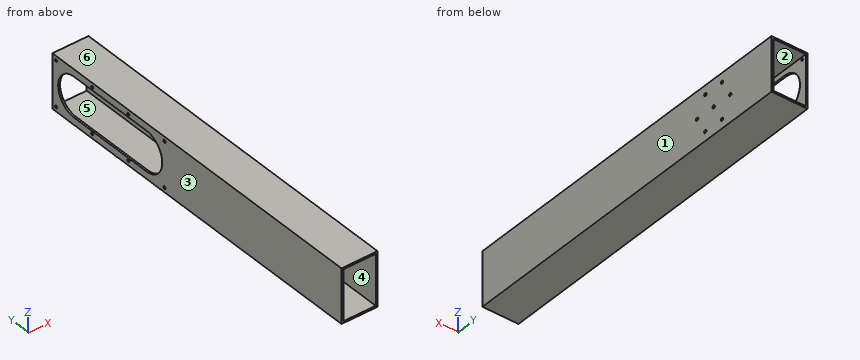
from build123d import *

# Parameters (mm, degrees)
SKETCH1_W                         = 40
SKETCH1_H                         = 60
SKETCH1_W_2                       = 36
SKETCH1_H_2                       = 56
BOSS_EXTRUDE1_DEPTH               = 400
M3_CLEARANCE_HOLE1_D              = 3.4
CUT_EXTRUDE1_DEPTH                = 3
TAP_DRILL_FOR_M3_TAP1_D           = 2.5
TAP_DRILL_FOR_M3_TAP1_DEPTH       = 2
TAP_DRILL_FOR_M3_TAP1_CSINK_D     = 3
TAP_DRILL_FOR_M3_TAP1_CSINK_ANGLE = 90


with BuildPart() as part:
    # Sketch1 → Boss-Extrude1 (new body)
    with BuildSketch(Plane(origin=(0, 0, 0), x_dir=(1, 0, 0), z_dir=(0, 1, 0))):
        with Locations((20, 30)):
            Rectangle(SKETCH1_W, SKETCH1_H)
        with Locations((20, 30)):
            Rectangle(SKETCH1_W_2, SKETCH1_H_2, mode=Mode.SUBTRACT)
    extrude(amount=BOSS_EXTRUDE1_DEPTH)

    # M3 Clearance Hole1 (through all)
    with Locations(Plane(origin=(40, 0, 0), x_dir=(0, 0, -1), z_dir=(1, 0, 0))):
        with Locations((30, 320), (30, 343), (49.918584287, 331.5), (49.918584287, 308.5), (30, 297), (10.081415713, 308.5), (10.081415713, 331.5)):
            Hole(M3_CLEARANCE_HOLE1_D / 2)

    # Sketch4 → Cut-Extrude1 (cut)
    with BuildSketch(Plane.ZY):
        with BuildLine():
            Line((-52, 270), (-52, 370))
            ThreePointArc((-52, 370), (-30, 392), (-8, 370))
            Line((-8, 370), (-8, 270))
            ThreePointArc((-8, 270), (-30, 248), (-52, 270))
        make_face()
    extrude(amount=-CUT_EXTRUDE1_DEPTH, mode=Mode.SUBTRACT)

    # Tap Drill for M3 Tap1
    with Locations(Plane.ZY):
        with Locations((-5, 245), (-55, 395), (-55, 245), (-55, 345), (-55, 295), (-5, 395), (-5, 345), (-5, 295)):
            CounterSinkHole(TAP_DRILL_FOR_M3_TAP1_D / 2, TAP_DRILL_FOR_M3_TAP1_CSINK_D / 2, depth=TAP_DRILL_FOR_M3_TAP1_DEPTH, counter_sink_angle=TAP_DRILL_FOR_M3_TAP1_CSINK_ANGLE)


solid = part.part
Build history of the part. All positions in model axes, mm. Face numbers are marked on the shaded views. A direction names the side the tool comes from. Coordinates: 2 decimals unless noted, no trailing zeros. Order: outer loops, then holes, each group sorted by start corner. A loop starts at its lowest first (then second) coordinate and runs counter-clockwise, first axis right, second up. Notation, with made-up numbers: (71, -3) -> (128, -3) arc R10 cw to (128, 11) -> close; hole circle Ø9 at (-39.5, -7.75). An arc over 180 degrees is marked (long way). One line per item, written item: value.
(1) Slice it at C-C, the plane z = -44. List the corners of the cut face in (x, y), plus the area to 3 significant figures.
Checked values:
outline: (0, 0) -> (2, 0) -> (2, 253.03) -> (0, 253.03) -> close; (0, 386.97) -> (2, 386.97) -> (2, 400) -> (0, 400) -> close; (38, 0) -> (40, 0) -> (40, 400) -> (38, 400) -> close
area: 1,330 mm2
(2) Drop a flat-ended pin along its axis: pin 1 Ø4.5 at (y, z) = (343, -30) entering from -X. Give the stop position or say it passes through.
Checked values:
pin 1: x = 38
(3) Tool access for the marked faces 1 and 2: list every direction of +Z, -Z, +X, -X, +Y, -Y with a clear straight run to the whole face (end or side of a thin tool).
Checked values:
face 1: +Z, -Z, +X, +Y, -Y
face 2: +Y, -Y
(4) Mould opens along Z. For the marked faces 3, 4, 5 and 6 say: pulls with the +Z half, pulls with the -Z half, needs draft (parallel to the pull), parting line crosses it, or undercut.
Checked values:
face 3: needs draft
face 4: undercut
face 5: undercut
face 6: pulls with the +Z half
(5) Probe line 1 (Y direction, x = 1.05, z = -5); line 2 (Z direction, x = 39, y = 308.5); line 3 (Z direction, x = 0.75, y = 395). List the from-to ranges inside material, lowest first. Write a range as [from, to].
Checked values:
line 1: [0, 243.75], [246.25, 293.75], [296.25, 343.75], [346.25, 393.75], [396.25, 400]
line 2: [-60, -51.62], [-48.22, -11.78], [-8.38, 0]
line 3: [-60, -56.25], [-53.75, -6.25], [-3.75, 0]
(6) Slice it at B-B, the plane x = 34.5. List the corners of the cut face in (y, z).
Checked values:
outline: (0, -60) -> (400, -60) -> (400, -58) -> (0, -58) -> close; (0, -2) -> (400, -2) -> (400, 0) -> (0, 0) -> close
(7) Slice it at A-A, the plane y = 73. List the corners of the cut face in (x, z).
Checked values:
outline: (0, -60) -> (40, -60) -> (40, 0) -> (0, 0) -> close; hole (2, -58) -> (38, -58) -> (38, -2) -> (2, -2) -> close
